Source: CAD feature listing. Evaluate the final solid. Frame: model axes, mm. Coordinates: 2 decimals unless noted, no trailing zeros.
```python
from build123d import *

# Parameters (mm, degrees)
BOSS_EXTRUDE1_DEPTH        = 1246.6
SKETCH3_W                  = 131.331771
SKETCH3_H                  = 32.627886
AILERON_CHORD_DEPTH        = 1246.6
SKETCH4_W                  = 171.070003
SKETCH4_H                  = 1110.639097
AILERON_SPAN_DEPTH         = 10
AILERON_SPAN_DEPTH_BACK    = 10
SKETCH5_R                  = 1.5
AILERON_SPAR_HOLE_DEPTH    = 144.8
SKETCH6_RX                 = 4.241084
SKETCH6_RY                 = 2.380428
AILERON_LEADING_EDGE_DEPTH = 143.8


with BuildPart() as part:
    # Sketch2 → Boss-Extrude1 (new body)
    with BuildSketch(Plane.XY):
        with BuildLine():
            ThreePointArc((164, 0.098236), (164.077667, 0), (164, -0.098236))
            add(Edge.make_bspline(
                [(164, 0.098236), (163.453347, 0.227855), (162.360116, 0.487077), (160.720174, 0.874803), (159.080335, 1.261114), (156.894332, 1.771897), (154.161962, 2.401008), (150.881841, 3.137526), (147.601665, 3.856594), (144.321702, 4.559852), (141.041699, 5.246218), (137.761757, 5.915572), (134.481686, 6.566534), (131.201761, 7.199898), (127.921668, 7.813754), (124.641701, 8.409172), (121.361598, 8.98465), (118.081601, 9.541284), (114.801561, 10.078059), (111.521601, 10.595035), (108.241714, 11.090965), (104.961715, 11.562926), (101.681786, 12.010167), (98.401747, 12.429709), (95.121663, 12.8205), (91.841542, 13.181831), (88.561414, 13.51363), (85.281283, 13.815894), (82.001169, 14.088695), (78.721095, 14.331741), (75.441021, 14.543175), (72.160895, 14.719913), (68.880726, 14.859428), (65.600503, 14.959161), (62.320225, 15.016118), (59.03999, 15.033011), (55.759815, 15.012804), (52.479681, 14.959634), (49.199602, 14.875645), (45.919233, 14.766825), (42.638538, 14.618827), (39.357416, 14.416023), (36.075798, 14.141603), (32.793534, 13.779736), (29.511749, 13.311849), (26.230435, 12.736941), (22.948211, 12.059087), (19.663974, 11.271431), (16.378115, 10.351738), (13.092739, 9.27165), (10.358156, 8.239856), (8.178743, 7.269153), (6.527119, 6.423629), (4.860633, 5.419015), (3.322168, 4.246728), (2.16678, 3.134219), (1.284844, 2.240038), (0.724778, 1.586326), (0.356487, 1.023715), (0.176339, 0.655159), (0.061261, 0.337633), (-0.042912, -0.12114), (0.010077, -0.598533), (0.176199, -1.014078), (0.354673, -1.344525), (0.71711, -1.82624), (1.269773, -2.336775), (2.131754, -2.920204), (3.354944, -3.392789), (4.915318, -3.707167), (6.554156, -4.03305), (8.195339, -4.283516), (10.38227, -4.5154), (13.118625, -4.672653), (16.398858, -4.828476), (19.679494, -4.922127), (22.959844, -4.966534), (26.240095, -4.967885), (29.520218, -4.932841), (32.800258, -4.868949), (36.080251, -4.782672), (39.360206, -4.679002), (42.64013, -4.562992), (45.920051, -4.439945), (49.199963, -4.314096), (52.479955, -4.190749), (55.759981, -4.070022), (59.039983, -3.95008), (62.320004, -3.83127), (65.600009, -3.712064), (68.880009, -3.592327), (72.16001, -3.47216), (75.439998, -3.351295), (78.720004, -3.230701), (81.999996, -3.109715), (85.279997, -2.989046), (88.559997, -2.868485), (91.84, -2.748159), (95.12, -2.627768), (98.4, -2.5074), (101.68, -2.387008), (104.960004, -2.266687), (108.24, -2.146109), (111.519996, -2.025503), (114.800005, -1.905264), (118.079995, -1.784568), (121.360005, -1.664353), (124.639995, -1.54365), (127.920005, -1.423438), (131.199995, -1.302734), (134.480005, -1.182522), (137.759995, -1.061818), (141.040005, -0.941606), (144.319995, -0.820902), (147.600005, -0.70069), (150.879995, -0.579986), (154.160005, -0.459776), (156.89333, -0.359182), (159.08, -0.278973), (160.72, -0.218763), (162.360004, -0.158632), (163.453334, -0.118368), (164, -0.098236)],
                knots=[0, 0, 0, 0, 0.005028, 0.010055, 0.015081, 0.020105, 0.030145, 0.040174, 0.050191, 0.060198, 0.070194, 0.08018, 0.090156, 0.100121, 0.110076, 0.12002, 0.129954, 0.139879, 0.149793, 0.159699, 0.169594, 0.17948, 0.189355, 0.199219, 0.209073, 0.218917, 0.228751, 0.238577, 0.248396, 0.258207, 0.268012, 0.277811, 0.287604, 0.297393, 0.307179, 0.316964, 0.326749, 0.336535, 0.346322, 0.356113, 0.365908, 0.375711, 0.385531, 0.395376, 0.405259, 0.415192, 0.425184, 0.435248, 0.445412, 0.455711, 0.466191, 0.471552, 0.477055, 0.482787, 0.488946, 0.494316, 0.497126, 0.500187, 0.502001, 0.503128, 0.50385, 0.50502, 0.507318, 0.507987, 0.509024, 0.510668, 0.513358, 0.515716, 0.519949, 0.524973, 0.529954, 0.534903, 0.539824, 0.54963, 0.559425, 0.569214, 0.579, 0.588784, 0.59857, 0.608356, 0.618144, 0.627933, 0.637724, 0.647515, 0.657307, 0.667099, 0.67689, 0.686681, 0.696472, 0.706263, 0.716054, 0.725846, 0.735637, 0.745428, 0.755219, 0.765011, 0.774802, 0.784593, 0.794384, 0.804176, 0.813967, 0.823758, 0.833549, 0.84334, 0.853132, 0.862923, 0.872714, 0.882505, 0.892297, 0.902088, 0.911879, 0.92167, 0.931461, 0.941253, 0.951044, 0.960835, 0.970626, 0.980418, 0.985313, 0.990209, 0.995104, 1, 1, 1, 1], degree=3))
        make_face()
    extrude(amount=BOSS_EXTRUDE1_DEPTH)

    # Sketch3 → Aileron chord (cut)
    with BuildSketch(Plane.XY.offset(1246.6)):
        with Locations((65.611782, 9.808584)):
            Rectangle(SKETCH3_W, SKETCH3_H)
    extrude(amount=-AILERON_CHORD_DEPTH, mode=Mode.SUBTRACT)

    # Sketch4 → Aileron span (cut, two sides)
    with BuildSketch(Plane(origin=(0, 0, 0), x_dir=(1, 0, 0), z_dir=(0, 1, 0))) as aileron_span_sk:
        with Locations((146.361743, -699.119548)):
            Rectangle(SKETCH4_W, SKETCH4_H)
    extrude(amount=AILERON_SPAN_DEPTH, mode=Mode.SUBTRACT)
    extrude(aileron_span_sk.sketch, amount=-AILERON_SPAN_DEPTH_BACK, mode=Mode.SUBTRACT)

    # Sketch5 → Aileron spar hole (cut, through all)
    with BuildSketch(Plane(origin=(0, 0, 0), x_dir=(-1, 0, 0), z_dir=(0, 0, -1))):
        with Locations((-137.277667, 2.94112)):
            Circle(SKETCH5_R)
    extrude(amount=-AILERON_SPAR_HOLE_DEPTH, mode=Mode.SUBTRACT)

    # Sketch6 → Aileron leading edge (add)
    with BuildSketch(Plane(origin=(0, 0, 0), x_dir=(-1, 0, 0), z_dir=(0, 0, -1))):
        with Locations(Location((-131.277667, 2.94112), (0, 0, 90))):
            Ellipse(SKETCH6_RX, SKETCH6_RY)
    extrude(amount=-AILERON_LEADING_EDGE_DEPTH)


solid = part.part
```
Q1. Pull-direction query (Y, two-part tool) for faces 1 (the cylindrical face through (138.776, 3.007, 70.893)), 2 (the flat face through (143, 2, 0)); classes: pulls with the +Y half, pulls with the -Y half, needs draft (parallel to the pull), parting line crosses it, or undercut.
Solutions:
face 1: undercut
face 2: needs draft
Q2. Pin query (flat end, axial travel): P1, Ø12, axis at x = 147.5, z = 33, coming from the +Y side; P2, Ø1, axis at y = 5.5, z = 75, coming from the -X side; P3, Ø10, axis at x = 157, z = 25.5, coming from the +Y side. Return the tip coordinate at first contact, or that it passes through.
Solutions:
P1: stops at y = 5.15
P2: stops at x = 129.2
P3: stops at y = 2.89
Q3. Material intervals for line 1 along Y through (x, z) = (135, 41.5); line 2 along Y through (x, z) = (136.5, 72); line 3 along Y through (x, z) = (160, 7.5), sorted ascending.
Solutions:
line 1: y = -1.16 to 6.46
line 2: y = -1.11 to 1.66, 4.22 to 6.17
line 3: y = -0.25 to 1.04
